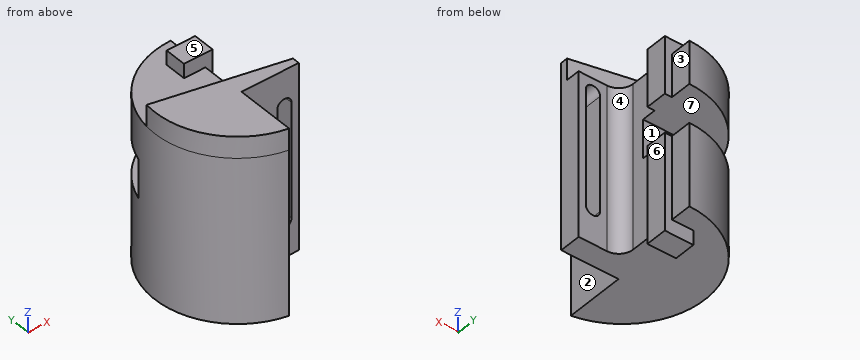
```python
from build123d import *

# Parameters (mm, degrees)
BOSS_EXTRUDE1_DEPTH      = 115
BOSS_EXTRUDE2_DEPTH      = 5
BOSS_EXTRUDE2_DEPTH_BACK = 15
CUT_EXTRUDE1_DEPTH       = 177.194640768
CUT_EXTRUDE1_DEPTH_BACK  = 177.194640768
SKETCH8_W                = 27
SKETCH8_H                = 40
BOSS_EXTRUDE3_DEPTH      = 15
CUT_EXTRUDE2_DEPTH       = 151.340654848


with BuildPart() as part:
    # Sketch1 → Boss-Extrude1 (new body)
    with BuildSketch(Plane.XY):
        with BuildLine():
            Line((0, 0), (0, 41.12760983))
            Line((0, 41.12760983), (40, 41.12760983))
            Line((40, 41.12760983), (40, 56.12760983))
            Line((40, 56.12760983), (20, 56.12760983))
            ThreePointArc((20, 56.12760983), (12.928932188, 59.056542018), (10, 66.12760983))
            Line((10, 66.12760983), (10, 114.62760983))
            ThreePointArc((10, 114.62760983), (-47.531489063, 61.896600381), (0, 0))
        make_face()
    extrude(amount=BOSS_EXTRUDE1_DEPTH)

    # Sketch5 → Boss-Extrude2 (add, two sides: drawn at the far end of the back side and taken through both)
    with BuildSketch(Plane(origin=(10, 0, 0), x_dir=(0, 0, -1), z_dir=(1, 0, 0)).offset(-BOSS_EXTRUDE2_DEPTH_BACK)):
        Polygon((0, 99.62760983), (10, 99.62760983), (10, 84.62760983), (-125, 84.62760983), (-125, 99.62760983), align=None)
    extrude(amount=BOSS_EXTRUDE2_DEPTH + BOSS_EXTRUDE2_DEPTH_BACK)

    # Sketch8 → Cut-Extrude1 (cut, two sides: drawn at the far end of the back side and taken through both)
    with BuildSketch(Plane(origin=(0, 0, 0), x_dir=(0, 0, -1), z_dir=(1, 0, 0)).offset(-CUT_EXTRUDE1_DEPTH_BACK)):
        with Locations((-71.5, 94.62760983)):
            Rectangle(SKETCH8_W, SKETCH8_H)
    extrude(amount=CUT_EXTRUDE1_DEPTH + CUT_EXTRUDE1_DEPTH_BACK, mode=Mode.SUBTRACT)

    # Sketch9 → Boss-Extrude3 (add)
    with BuildSketch(Plane.XY.offset(115)):
        with BuildLine():
            Line((40, 46.12760983), (-47.222231128, 64.66726738))
            ThreePointArc((-47.222231128, 64.66726738), (-36.638728081, 22.82042934), (0, 0))
            Line((0, 0), (0, 41.12760983))
            Line((0, 41.12760983), (40, 41.12760983))
            Line((40, 41.12760983), (40, 46.12760983))
        make_face()
    extrude(amount=BOSS_EXTRUDE3_DEPTH)

    # Sketch10 → Cut-Extrude2 (cut, through all)
    with BuildSketch(Plane(origin=(0, 56.12760983, 0), x_dir=(1, 0, 0), z_dir=(0, 1, 0))):
        with BuildLine():
            Line((25, -105), (25, -25))
            ThreePointArc((25, -25), (30, -20), (35, -25))
            Line((35, -25), (35, -105))
            ThreePointArc((35, -105), (30, -110), (25, -105))
        make_face()
    extrude(amount=-CUT_EXTRUDE2_DEPTH, mode=Mode.SUBTRACT)


solid = part.part
```
Verification items for the finished model (mm, model axes). Face numbers are marked on the shaded views. A direction names the side the tool comes from. Round coordinates to 2 decimals unless told otherwise and drop trailing zeros. Write each loop counter-clockwise with the first axis right and the second up, starting at its lowest first coordinate (ties: lowest second). Pieces come first, ordered by that corner, then holes. Notation, with made-up numbers: (77.5, 83) -> (124.5, 83) arc R20 ccw to (124.5, 120) -> close; hole circle Ø7 at (9.25, -22.75). An arc over 180 degrees is marked (long way). Write each question's results on one line, items separated by ' | '.
Q1. Access from +Z, -Z, +X, -X, +Y, -Y to the whole of each face (thin tool, end or side, straight path). Record for the marked faces 1, 2, 3 and 4.
Derived:
face 1: +X, -X, +Y | face 2: +Z, -Z, +X, -Y | face 3: +Z, -Z, +X, +Y | face 4: +Z, -Z, +X
Q2. Sectioned sample at C-C, the plane z = 9.5. Record the boundary of the cut face in (x, y).
Derived:
outline: (0, 0) -> (0, 41.13) -> (40, 41.13) -> (40, 56.13) -> (20, 56.13) arc R10 cw to (10, 66.13) -> (10, 84.63) -> (15, 84.63) -> (15, 99.63) -> (10, 99.63) -> (10, 114.63) arc R57.75 ccw to start
Q3. Thickness scan on probe 1 along Z at (x, y) = (-12, 88); probe 2 along Y at (x, z) = (22, 102); probe 3 along Z at (x, y) = (-33, 69). Record the ranges inside material, lowest first.
Derived:
probe 1: z = 0 to 58, 85 to 115 | probe 2: y = 41.13 to 56.13 | probe 3: z = 0 to 115
Q4. Sectioned sample at D-D, the plane x = 12.5. Record the boundary of the cut face in (y, z).
Derived:
outline: (41.13, 0) -> (59.51, 0) -> (59.51, 115) -> (51.97, 115) -> (51.97, 130) -> (41.13, 130) -> close; (84.63, -10) -> (99.63, -10) -> (99.63, 58) -> (84.63, 58) -> close; (84.63, 85) -> (99.63, 85) -> (99.63, 125) -> (84.63, 125) -> close
Q5. Sectioned sample at B-B, the plane x = 30. Record the boundary of the cut face in (y, z), and give its area (3 significant figures).
Derived:
outline: (41.13, 0) -> (56.13, 0) -> (56.13, 20) -> (41.13, 20) -> close; (41.13, 110) -> (56.13, 110) -> (56.13, 115) -> (48.25, 115) -> (48.25, 130) -> (41.13, 130) -> close | area: 482 mm²
Q6. Sectioned sample at A-A, the plane z = 88. Record the boundary of the cut face in (x, y).
Derived:
outline: (0, 0) -> (0, 41.13) -> (25, 41.13) -> (25, 56.13) -> (20, 56.13) arc R10 cw to (10, 66.13) -> (10, 84.63) -> (15, 84.63) -> (15, 99.63) -> (10, 99.63) -> (10, 114.63) arc R57.75 ccw to start; (35, 41.13) -> (40, 41.13) -> (40, 56.13) -> (35, 56.13) -> close
Q7. Go/stop test with flat-tipped pins: pin 1 Ø16 at (x, z) = (8.5, 16) entering from -Y; pin 2 Ø10 at (x, z) = (1, 99) entering from -Y; pin 3 Ø2 at (x, y) = (-9, 41) entering from -Z. Record where each tip stops, or that it passes through.
Derived:
pin 1: stops at y = 41.13 | pin 2: stops at y = 0 | pin 3: stops at z = 0
Q8. Draft check along Z on the marked faces 5, 6 and 7. Enter one of: released by +Z, released by -Z, zero draft, split by the parting line, or undercut.
Derived:
face 5: released by +Z | face 6: zero draft | face 7: undercut
